Verification items for the finished model (mm, model axes). A direction names the side the tool comes from. Give positions to 0.01 mm unless a question says otherwise; leave off trailing zeros. Order: outer loops, then holes, each group sorted by start corner. A loop starts at its lowest first (then second) coordinate and runs counter-clockwise, first axis right, second up. Notation, with made-up numbers: (-10, 9.25) -> (18, 9.25) arc R6 cw to (18, 19.25) -> close; hole circle Ø7 at (20, -13.5). An arc over 180 degrees is marked (long way). Write each question's results on one line, items separated by ' | '. Start each with the question number.
1. Material ranges on L1, parallel to Z at x = 4, y = 15; L2, parallel to Y at x = 59, z = 12; L3, parallel to X at y = 39, z = 31.5, recorded low to high. Write a range as from..to.
2. Depth check by flat-ended pin: pin 1 Ø3 at (x, y) = (23, 27) entering from +Z; pin 2 Ø4 at (y, z) = (33, 28.5) entering from -X. Enter the tip coordinate at first touch or a pass-through.
3. Cross-section at B-B, the plane y = 12. Enter the section's corners in (x, z).
4. Cross-section at A-A, the plane x = 48. Enter the section's corners in (y, z).
5. Cross-section at D-D, the plane x = 23.5. Enter the section's corners in (y, z).
6. Set-up check for faces 1 (the face through (60.473, 30.815, 30.514)), 2 (the face through (32, 45, 14)), 3 (the face through (58, 39, 28)): record each of +Z, -Z, +X, -X, +Y, -Y from which the full face is reachable in a straight line by a thin tool's end or side.
7. Cross-section at C-C, the plane y = 20. Enter the section's corners in (x, z).
from build123d import *

# Parameters (mm, degrees)
BOSS_EXTRUDE1_DEPTH = 28
FILLET1_R           = 3
SKETCH4_R           = 12.5
BOSS_EXTRUDE3_DEPTH = 5


with BuildPart() as part:
    # Sketch3 → Boss-Extrude1 (new body)
    with BuildSketch(Plane.XY):
        with BuildLine():
            Line((5, 0), (58, 0))
            ThreePointArc((58, 0), (61.535533906, 1.464466094), (63, 5))
            Line((63, 5), (63, 40))
            ThreePointArc((63, 40), (61.535533906, 43.535533906), (58, 45))
            Line((58, 45), (5, 45))
            ThreePointArc((5, 45), (1.464466094, 43.535533906), (0, 40))
            Line((0, 40), (0, 5))
            ThreePointArc((0, 5), (1.464466094, 1.464466094), (5, 0))
        make_face()
    extrude(amount=BOSS_EXTRUDE1_DEPTH)

    # Fillet1
    fillet1_edges = [part.edges().sort_by_distance(p)[0] for p in [
        (63, 22.5, 0),
        (61.535533906, 1.464466094, 0),
        (31.5, 0, 0),
        (1.464466094, 1.464466094, 0),
        (61.535533906, 1.464466094, 28),
        (63, 22.5, 28),
        (61.535533906, 43.535533906, 28),
        (31.5, 45, 28),
        (1.464466094, 43.535533906, 28),
        (0, 22.5, 28),
        (1.464466094, 1.464466094, 28),
        (0, 22.5, 0),
        (31.5, 0, 28),
        (1.464466094, 43.535533906, 0),
        (31.5, 45, 0),
        (61.535533906, 43.535533906, 0),
    ]]
    fillet(fillet1_edges, radius=FILLET1_R)

    # Sketch4 → Boss-Extrude3 (add, symmetric)
    with BuildSketch(Plane.XY.offset(28)):
        with Locations(Location((48, 30, 0), (0, 0, 106.260204708))):
            Circle(SKETCH4_R)
    extrude(amount=BOSS_EXTRUDE3_DEPTH, both=True)


solid = part.part
Results below:
1) L1: z = 0..28 | L2: y = 0.1..44.9 | L3: x = 39.33..56.67
2) pin 1: stops at z = 28 | pin 2: stops at x = 0.4
3) outline: (0, 3) arc R3 ccw to (3, 0) -> (60, 0) arc R3 ccw to (63, 3) -> (63, 25) arc R3 ccw to (60, 28) -> (3, 28) arc R3 ccw to (0, 25) -> close
4) outline: (0, 3) arc R3 ccw to (3, 0) -> (42, 0) arc R3 ccw to (45, 3) -> (45, 25) arc R3 ccw to (42.5, 27.96) -> (42.5, 33) -> (17.5, 33) -> (17.5, 28) -> (3, 28) arc R3 ccw to (0, 25) -> close
5) outline: (0, 3) arc R3 ccw to (3, 0) -> (42, 0) arc R3 ccw to (45, 3) -> (45, 25) arc R3 ccw to (42, 28) -> (3, 28) arc R3 ccw to (0, 25) -> close
6) face 1: +Z | face 2: +Z, -Z, +X, -X, +Y | face 3: +Z, +X, +Y
7) outline: (0, 3) arc R3 ccw to (3, 0) -> (60, 0) arc R3 ccw to (63, 3) -> (63, 25) arc R3 ccw to (60, 28) -> (55.5, 28) -> (55.5, 33) -> (40.5, 33) -> (40.5, 28) -> (3, 28) arc R3 ccw to (0, 25) -> close
